from build123d import *

# Parameters (mm, degrees)
SKETCH1_W           = 0.6
SKETCH1_H           = 1.7
BOSS_EXTRUDE1_DEPTH = 0.4
FILLET1_R           = 1
SKETCH3_W           = 0.6
SKETCH3_H           = 0.9
SKETCH3_H_2         = 1
CUT_EXTRUDE2_DEPTH  = 0.05


with BuildPart() as part:
    # Sketch1 → Boss-Extrude1 (new body)
    with BuildSketch(Plane(origin=(0, 0, 0), x_dir=(1, 0, 0), z_dir=(0, 1, 0))):
        Polygon((0, 0), (7, 0), (7, 7), (0.3, 7), (0.3, 5), (0, 5), (0, 3), (0.3, 3), (0.3, 1.5), (0, 1.5), align=None)
        with Locations((4.7, 5.15)):
            Rectangle(SKETCH1_W, SKETCH1_H, mode=Mode.SUBTRACT)
        with Locations((6.2, 1.75)):
            Rectangle(SKETCH1_W, SKETCH1_H, mode=Mode.SUBTRACT)
    extrude(amount=BOSS_EXTRUDE1_DEPTH)

    # Fillet1
    fillet1_edges = [part.edges().sort_by_distance(p)[0] for p in [
        (0.3, 0.2, -7),
        (7, 0.2, -7),
        (7, 0.2, 0),
    ]]
    fillet(fillet1_edges, radius=FILLET1_R)

    # Sketch3 → Cut-Extrude2 (cut)
    with BuildSketch(Plane(origin=(0, 0.4, 0), x_dir=(1, 0, 0), z_dir=(0, 1, 0))):
        with BuildLine():
            Line((1.5, 0), (1.5, 7))
            Line((1.5, 7), (1.3, 7))
            ThreePointArc((1.3, 7), (0.592893219, 6.707106781), (0.3, 6))
            Line((0.3, 6), (0.3, 5))
            Line((0.3, 5), (0, 5))
            Line((0, 5), (0, 3))
            Line((0, 3), (0.3, 3))
            Line((0.3, 3), (0.3, 1.5))
            Line((0.3, 1.5), (0, 1.5))
            Line((0, 1.5), (0, 0))
            Line((0, 0), (1.5, 0))
        make_face()
        with Locations((6.2, 0.45)):
            Rectangle(SKETCH3_W, SKETCH3_H)
        Polygon((4.4, 4.3), (5, 4.3), (5.9, 4.3), (5.9, 7), (5.9, 7.268876882), (6.5, 7.268876882), (6.5, 7), (6.5, 4.3), (6.5, 3.7), (6.5, 2.6), (5.9, 2.6), (5.9, 3.7), (4.4, 3.7), align=None)
        with Locations((4.7, 6.5)):
            Rectangle(SKETCH3_W, SKETCH3_H_2)
    extrude(amount=-CUT_EXTRUDE2_DEPTH, mode=Mode.SUBTRACT)


solid = part.part
CAD build for the part. Positions are in the model's coordinates, mm. Round coordinates to 2 decimals unless told otherwise and drop trailing zeros. Order: outer loops, then holes, each group sorted by start corner. A loop starts at its lowest first (then second) coordinate and runs counter-clockwise, first axis right, second up. Notation, with made-up numbers: M 63,-7.5 L 110,-7.5 A32 cw 110,26.5 Z; hole C 65,69 d4. An arc over 180 degrees is marked long. Use one line per item in the form item = value.
Q1. Saw through at C-C on x = 6.25. Give the cut face in (y, z).
Recorded:
outline = M 0,-6.97 L 0.35,-6.97 L 0.35,-2.6 L 0,-2.6 Z; M 0,-0.9 L 0.35,-0.9 L 0.35,-0.03 L 0,-0.03 Z
Q2. Saw through at A-A on z = -1.25. Give the cut face in (x, y).
Recorded:
outline = M 0,0 L 5.9,0 L 5.9,0.4 L 1.5,0.4 L 1.5,0.35 L 0,0.35 Z; M 6.5,0 L 7,0 L 7,0.4 L 6.5,0.4 Z
Q3. Probe L1, parallel to X at y = 0.05, z = -4.5; L2, parallel to Z at x = 4.75, y = 0.3; L3, parallel to Y at x = 0.5, z = -1.5. List the from-to ranges inside material, lowest first.
Recorded:
L1 = 0 to 4.4, 5 to 7
L2 = -7 to -6, -4.3 to 0
L3 = 0 to 0.35
Q4. Saw through at D-D on z = -4.75. Give the cut face in (x, y), then the cut area to 4 significant figures.
Recorded:
outline = M 0,0 L 4.4,0 L 4.4,0.4 L 1.5,0.4 L 1.5,0.35 L 0,0.35 Z; M 5,0 L 7,0 L 7,0.4 L 6.5,0.4 L 6.5,0.35 L 5.9,0.35 L 5.9,0.4 L 5,0.4 Z
area = 2.455 mm^2
Q5. Saw through at B-B on y = 0.1. Give the cut face in (x, z).
Recorded:
outline = M 0,-5 L 0.3,-5 L 0.3,-6 A1 ccw 1.3,-7 L 6,-7 A1 ccw 7,-6 L 7,-1 A1 ccw 6,0 L 0,0 L 0,-1.5 L 0.3,-1.5 L 0.3,-3 L 0,-3 Z; hole M 4.4,-6 L 5,-6 L 5,-4.3 L 4.4,-4.3 Z; hole M 5.9,-2.6 L 6.5,-2.6 L 6.5,-0.9 L 5.9,-0.9 Z
Q6. Two-plate mould, pull along X, no slides. Class faces 1 (the cylindrical face through (6.699, 0.203, -0.285)), 2 (the cylindrical face through (0.601, 0.177, -6.715)), 3 (the flat face through (6.2, 0.35, -4.8)), 4 (the flat face through (1, 0.35, -4)): +X half, -X half, draft (parallel to the pull), parting line (faces both ways), or undercut.
Recorded:
face_1 = +X half
face_2 = -X half
face_3 = undercut
face_4 = draft
